Here's how the part is built. I have some questions about the finished solid (model axes, mm). Face numbers are marked on the shaded views. A direction names the side the tool comes from. Give positions to 0.01 mm unless a question says otherwise; leave off trailing zeros. Loops run counter-clockwise (first coordinate to the right, second up) from the corner with the lowest first, then second, coordinate; pieces in that order, holes last.
Q1. Suppose I cut it at C-C (x = 0.5). List the corners of the cut face in (y, z) for me, and give its area (3 significant figures).
Q2. Suppose I cut it at B-B (z = -4). List the corners of the cut face in (x, y) for me.
Q3. Suppose I cut it at D-D (y = -3). List the corners of the cut face in (x, z) for me, and give its area (3 significant figures).
Q4. For the marked faces 1, 2, 3 and 4, which set-ups out of +Z, -Z, +X, -X, +Y, -Y let a thin tool reach every point of the face, with its end or its side?
Q5. Thinking about a two-plate mould opening in Z: for the marked faces 5 and 6, which applies, pulls with the +Z half, pulls with the -Z half, needs draft (parallel to the pull), parting line crosses it, or undercut?
Q6. I'm going to push flat-ended pins straight in: P1, Ø1.5, axis at x = -12, z = -7, coming from the -Y side; P2, Ø4, axis at x = -35, z = 14, coming from the -Y side; P3, Ø5, axis at x = -4.5, z = 10, coming from the -Y side; P4, Ø2.5, axis at x = -35, z = -14, coming from the +Y side. Where does each tip first touch, or does it pass through?
Q7. Suppose I cut it at A-A (x = -35). List the corners of the cut face in (y, z) for me.
Q8. I need wall thicknesses on probe 1 along Z at (x, y) = (-35, -1.4); probe 2 along X at (y, z) = (-0.9, -14); probe 3 along X at (y, z) = (-1.75, -12). Which ranges of each line are inside material? Lowest first, please.
```python
from build123d import *

# Parameters (mm, degrees)
SKETCH1_W               = 60
SKETCH1_H               = 35
BOSS_EXTRUDE1_DEPTH     = 8
CUT_EXTRUDE1_DEPTH      = 1
CUT_EXTRUDE1_DEPTH_BACK = 61
FILLET1_R               = 2
SKETCH3_W               = 20
SKETCH3_H               = 2
CUT_EXTRUDE2_DEPTH      = 36
SKETCH5_W               = 35
SKETCH5_H               = 2
BOSS_EXTRUDE2_DEPTH     = 10
SKETCH6_R               = 1.6
CUT_EXTRUDE3_DEPTH      = 10


with BuildPart() as part:
    # Sketch1 → Boss-Extrude1 (new body)
    with BuildSketch(Plane(origin=(0, 0, 0), x_dir=(1, 0, 0), z_dir=(0, 1, 0))):
        Rectangle(SKETCH1_W, SKETCH1_H)
    extrude(amount=-BOSS_EXTRUDE1_DEPTH)

    # Sketch2 → Cut-Extrude1 (cut, two sides)
    with BuildSketch(Plane(origin=(30, 0, 0), x_dir=(0, 0, -1), z_dir=(1, 0, 0))) as cut_extrude1_sk:
        Polygon((-12.5, -5), (-17.5, -8), (0, -8), (0, -5), align=None)
        Polygon((0, -5), (0, -8), (17.5, -8), (12.5, -5), align=None)
    extrude(amount=CUT_EXTRUDE1_DEPTH, mode=Mode.SUBTRACT)
    extrude(cut_extrude1_sk.sketch, amount=-CUT_EXTRUDE1_DEPTH_BACK, mode=Mode.SUBTRACT)

    # Fillet1
    fillet1_edges = [part.edges().sort_by_distance(p)[0] for p in [
        (0, -8, -17.5),
        (0, -5, 12.5),
        (0, -5, -12.5),
        (0, -8, 17.5),
    ]]
    fillet(fillet1_edges, radius=FILLET1_R)

    # Sketch3 → Cut-Extrude2 (cut, through all)
    with BuildSketch(Plane.XY.offset(17.5)):
        with Locations((-15, -1)):
            Rectangle(SKETCH3_W, SKETCH3_H)
        with Locations((15, -1)):
            Rectangle(SKETCH3_W, SKETCH3_H)
    extrude(amount=-CUT_EXTRUDE2_DEPTH, mode=Mode.SUBTRACT)

    # Sketch5 → Boss-Extrude2 (add)
    with BuildSketch(Plane.ZY.offset(30)):
        with Locations((0, -1)):
            Rectangle(SKETCH5_W, SKETCH5_H)
    boss_extrude2 = extrude(amount=BOSS_EXTRUDE2_DEPTH)

    # Mirror1: Boss-Extrude2 across plane
    add(boss_extrude2.mirror(Plane(origin=(0, 0, 0), x_dir=(0, 0, 1), z_dir=(1, 0, 0))))

    # Sketch6 → Cut-Extrude3 (cut)
    with BuildSketch(Plane(origin=(0, 0, 0), x_dir=(1, 0, 0), z_dir=(0, 1, 0))):
        with Locations((-35, 14)):
            Circle(SKETCH6_R)
        with Locations((35, 14)):
            Circle(SKETCH6_R)
        with Locations((35, -14)):
            Circle(SKETCH6_R)
        with Locations((-35, -14)):
            Circle(SKETCH6_R)
    extrude(amount=-CUT_EXTRUDE3_DEPTH, mode=Mode.SUBTRACT)


solid = part.part
```
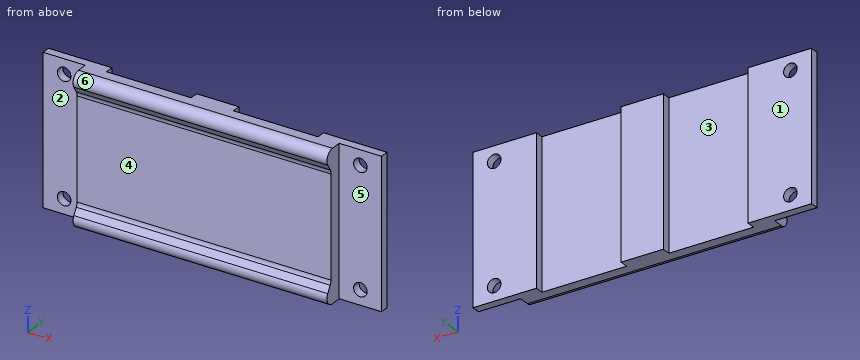
Solutions:
1. outline: (-6.18, -14.47) arc R2 ccw to (-4.47, -17.5) - (0, -17.5) - (0, 17.5) - (-4.47, 17.5) arc R2 ccw to (-6.18, 14.47) - (-5.29, 12.98) arc R2 cw to (-5, 11.95) - (-5, -11.95) arc R2 cw to (-5.29, -12.98) - close
1. area: 184 mm2
2. outline: (-40, -2) - (-30, -2) - (-30, -5) - (30, -5) - (30, -2) - (40, -2) - (40, 0) - (25, 0) - (25, -2) - (5, -2) - (5, 0) - (-5, 0) - (-5, -2) - (-25, -2) - (-25, 0) - (-40, 0) - close
3. outline: (-30, -17.5) - (30, -17.5) - (30, 17.5) - (-30, 17.5) - close
3. area: 2,100 mm2
4. face 1: +Z, -Z, +X, -X, +Y
4. face 2: +Z, -Z, -X, -Y
4. face 3: +Z, -Z, +Y
4. face 4: +X, -X, -Y
5. face 5: needs draft
5. face 6: undercut
6. P1: stops at y = -5
6. P2: stops at y = -2
6. P3: stops at y = -5.08
6. P4: passes through
7. outline: (-2, -17.5) - (0, -17.5) - (0, -15.6) - (-2, -15.6) - close; (-2, -12.4) - (0, -12.4) - (0, 12.4) - (-2, 12.4) - close; (-2, 15.6) - (0, 15.6) - (0, 17.5) - (-2, 17.5) - close
8. probe 1: z = -17.5 to -15.6, -12.4 to 12.4, 15.6 to 17.5
8. probe 2: x = -40 to -36.6, -33.4 to -25, -5 to 5, 25 to 33.4, 36.6 to 40
8. probe 3: x = -40 to -25, -5 to 5, 25 to 40
